```python
from build123d import *

# Parameters (mm, degrees)
SKETCH1_W                = 76
SKETCH1_H                = 35
BOSS_EXTRUDE1_DEPTH      = 30
BOSS_EXTRUDE2_DEPTH      = 8
BOSS_EXTRUDE2_DEPTH_BACK = 3
SKETCH2_W                = 10
SKETCH2_H                = 18


with BuildPart() as part:
    # Sketch1 → Boss-Extrude1 (new body)
    with BuildSketch(Plane.XY):
        Rectangle(SKETCH1_W, SKETCH1_H)
    extrude(amount=BOSS_EXTRUDE1_DEPTH)

    # Sketch2 → Boss-Extrude2 (add, two sides: drawn at the far end of the back side and taken through both)
    with BuildSketch(Plane(origin=(0, 17.5, 0), x_dir=(1, 0, 0), z_dir=(0, 1, 0)).offset(-BOSS_EXTRUDE2_DEPTH_BACK)):
        with Locations((-37, -15)):
            Rectangle(SKETCH2_W, SKETCH2_H)
    extrude(amount=BOSS_EXTRUDE2_DEPTH + BOSS_EXTRUDE2_DEPTH_BACK)


solid = part.part
```
Source: CAD feature listing. Evaluate the final solid. Frame: model axes, mm. A direction names the side the tool comes from. Coordinates: 2 decimals unless noted, no trailing zeros. Loops run counter-clockwise (first coordinate to the right, second up) from the corner with the lowest first, then second, coordinate; pieces in that order, holes last. Notation, with made-up numbers: (10.25, 45) -> (33.25, 45) arc R29 ccw to (33.25, 71) -> close; hole circle Ø9 at (76, 28.25). An arc over 180 degrees is marked (long way). One line per item, written item: value. Start each with the question number.
Q1. Section query C-C, the plane y = 13.5. Return the cut outline in (x, z).
Q2. Set-up query: faces 1 (the face through (-32, 21, 15)), 2 (the face through (-1, -17.5, 15)), 3 (the face through (-40, 14.5, 15)). Return all of +Z, -Z, +X, -X, +Y, -Y with unobstructed straight access to the full face (end or side cutting, diameter ignored); none if empty.
Q3. Line query: line 1 along Y through (x, z) = (-25, 10.75); line 2 along X through (y, z) = (-7.5, 5.25). Output: solid intervals per line, ascending.
Q4. Section query B-B, the plane x = 19.5. Return the cut outline in (y, z), and give its area (3 significant figures).
Q5. Section query A-A, the plane z = 20.25. Return the cut outline in (x, y).
Q6. Contact query for flat-ended pins moving along their axis: P1, Ø12, axis at x = 22.5, z = 6, coming from the +Y side; P2, Ø8, axis at x = -35, y = 22.5, coming from the -Z side; P3, Ø9, axis at y = -1.5, z = 17.5, coming from the -X side. Output: stop coordinate, or through.
Results:
1. outline: (-38, 0) -> (38, 0) -> (38, 30) -> (-38, 30) -> close
2. face 1: +Z, -Z, +X, +Y
2. face 2: +Z, -Z, +X, -X, -Y
2. face 3: +Z, -Z, -X, -Y
3. line 1: -17.5 to 17.5
3. line 2: -38 to 38
4. outline: (-17.5, 0) -> (17.5, 0) -> (17.5, 30) -> (-17.5, 30) -> close
4. area: 1,050 mm^2
5. outline: (-42, 14.5) -> (-38, 14.5) -> (-38, -17.5) -> (38, -17.5) -> (38, 17.5) -> (-32, 17.5) -> (-32, 25.5) -> (-42, 25.5) -> close
6. P1: y = 17.5
6. P2: z = 6
6. P3: x = -38
